For this review, take the finished solid that the model builds, in its own axes (mm). A direction names the side the tool comes from. Coordinates: 2 decimals unless noted, no trailing zeros. Order: outer loops, then holes, each group sorted by start corner. A loop starts at its lowest first (then second) coordinate and runs counter-clockwise, first axis right, second up. Notation, with made-up numbers: (34.25, 13.5) - (44.25, 13.5) arc R32 cw to (44.25, 46.5) - close; hole circle Ø6 at (10, 28). An arc over 180 degrees is marked (long way). One line per item, written item: value. Start each with the question number.
(1) Consider section B-B on y = 2.25. Write out the cut boundary in (x, z).
(2) Clearance check with flat-ended pins moving along their axes: pin 1 (9 mm diameter, centred on y = 10, z = -43.5, fed in from +X); pin 2 (1.5 mm diameter, centred on y = 13.5, z = 43.5, fed in from +X); pin 3 (1 mm diameter, centred on x = 22.5, y = 5, fed in from -Z); pin 4 (2.5 mm diameter, centred on x = -12.83, z = 39.86, fed in from -Y). State where each tip first meets the part, or that it passes through.
(3) Consider section A-A on z = 0. Write out the cut boundary in (x, y), then the cut area to 3 significant figures.
(4) Mouldability with a two-part tool opening along Z and no side actions: class faces 1 (the cylindrical face through (12.465, 7.395, 56.133)), 2 (the flat face through (1, 0, 1)), 3 (the cylindrical face through (0.01, 12.9, 31.91)) as released by +Z, released by -Z, zero draft, split by the parting line, or undercut.
(5) For faces 4 (the flat face through (0, 15, 39)), 5 (the flat face through (3, 9, 41)), list the 3-axis set-ups (+Z, -Z, +X, -X, +Y, -Y) from which the entire face can be reached by the end or side of a thin tool; tool diameter is ignored.
(6) To check wall thickness, follow line 1 along X through (y, z) = (5.75, 43); line 2 along X through (y, z) = (12, -46); line 3 along Y through (x, z) = (-5.5, -19). State the ranges of each line that lie inside material, in increasing order.
Autodesk Inventor part; units mm, degrees
ref_plane "YZ Plane" through (0, 0, 0) normal (1, 0, 0) x (0, 1, 0)
ref_plane "XZ Plane" through (0, 0, 0) normal (0, 1, 0) x (-1, 0, 0)
ref_plane "XY Plane" through (0, 0, 0) normal (0, 0, 1) x (1, 0, 0)
sketch "Sketch1" plane through (0, 0, 0) normal (0, 1, 0) x (-1, 0, 0)
  circle A0 centre (0, 0) radius 57.5
  dimension "d0" = 115
extrude "Extrusion1" add sketch "Sketch1" along normal blind 15
sketch "Sketch2" plane through (0, 15, 0) normal (0, 1, 0) x (1, 0, 0)
  circle A0 centre (0, 0) radius 57.5 construction
  circle A1 centre (0, 0) radius 50
  dimension "d3" = 100
extrude "Extrusion2" cut sketch "Sketch2" against normal blind 10
sketch "Sketch3" plane through (0, 5, 0) normal (0, 1, 0) x (1, 0, 0)
  circle A0 centre (0, 0) radius 50 construction
  line L0 (-3, -49.9099) -> (-3, -29.9099)
  line L1 (-3, -29.9099) -> (3, -29.9099)
  line L2 (3, -29.9099) -> (3, -49.9099)
  circle A1 centre (0, 0) radius 50
  line L3 (0, 0) -> (-15.0126, 0) construction
  circle A2 centre (0, 0) radius 50 construction
  line L4 (-3, 49.9099) -> (-3, 29.9099)
  line L5 (-3, 29.9099) -> (3, 29.9099)
  line L6 (3, 29.9099) -> (3, 49.9099)
  circle A3 centre (0, 0) radius 50
  dimension "d6" = 20
  dimension "d7" = 3
  dimension "d8" = 6
extrude "Extrusion3" add sketch "Sketch3" along normal blind 10 contours L0 L1 L2 A1 | A1 L6 L5 L4
fillet "Fillet2" radius 7 2 edges at (0, 15, 29.9099) (0, 15, -29.9099)
fillet "Fillet3" radius 2 14 edges at (3, 12.9497, -31.9602) (3, 6.5, -29.9099) (3, 15, -43.4099) (-3, 12.9497, -31.9602) (-3, 6.5, -29.9099) (-3, 15, -43.4099) (-50, 15, 0) (50, 15, 0) (3, 12.9497, 31.9602) (3, 6.5, 29.9099) (3, 15, 43.4099) (-3, 12.9497, 31.9602) (-3, 6.5, 29.9099) (-3, 15, 43.4099)
thread "Thread1"
sketch "Sketch4" plane through (0, 5, 0) normal (0, 1, 0) x (1, 0, 0)
  circle A0 centre (-12.8327, -39.8572) radius 1
  dimension "d16" = 2
extrude "Extrusion4" cut sketch "Sketch4" against normal blind 10
properties part number "Capac" material "Glass"
Geometry check:
1. outline: circle Ø115 at (0, 0); hole circle Ø2 at (-12.83, 39.86)
2. pin 1: stops at x = 42.25
2. pin 2: stops at x = 38.45
2. pin 3: stops at z = -53.12
2. pin 4: stops at y = 0
3. outline: (-57.5, 0) - (57.5, 0) - (57.5, 15) - (52, 15) arc R2 ccw to (50, 13) - (50, 5) - (-50, 5) - (-50, 13) arc R2 ccw to (-52, 15) - (-57.5, 15) - close
3. area: 723 mm^2
4. face 1: split by the parting line
4. face 2: zero draft
4. face 3: undercut
5. face 4: +Z, -Z, +X, -X, +Y
5. face 5: +Y
6. line 1: x = -38.17 to -25.51, -3 to 3, 25.51 to 38.17
6. line 2: x = -34.5 to -19.6, -3 to 3, 19.6 to 34.5
6. line 3: y = 0 to 5
